Autodesk Fusion 360 part; units mm, degrees
sketch "Sketch1" plane through (0, 0, 0) normal (0, 0, 1) x (1, 0, 0)
  line L0 (-12.2461, -1.8602) -> (-7.8071, 9.2886)
  line L1 (-7.8071, 9.2886) -> (4.0675, 11.0187)
  line L2 (4.0675, 11.0187) -> (11.5031, 1.6)
  line L3 (11.5031, 1.6) -> (7.0641, -9.5488)
  line L4 (7.0641, -9.5488) -> (-4.8105, -11.2789)
  line L5 (-4.8105, -11.2789) -> (-12.2461, -1.8602)
  line L6 (-4.8105, -11.2789) -> (7.0641, -9.5488)
  line L7 (7.0641, -9.5488) -> (9.515, -26.3712)
  line L8 (9.515, -26.3712) -> (-2.3596, -28.1013)
  line L9 (-2.3596, -28.1013) -> (-4.8105, -11.2789)
  line L10 (7.0641, -9.5488) -> (11.5031, 1.6)
  line L11 (11.5031, 1.6) -> (27.2972, -4.6887)
  line L12 (27.2972, -4.6887) -> (22.8582, -15.8374)
  line L13 (22.8582, -15.8374) -> (7.0641, -9.5488)
  line L14 (11.5031, 1.6) -> (4.0675, 11.0187)
  line L15 (4.0675, 11.0187) -> (17.4107, 21.5524)
  line L16 (17.4107, 21.5524) -> (24.8463, 12.1337)
  line L17 (24.8463, 12.1337) -> (11.5031, 1.6)
  line L18 (4.0675, 11.0187) -> (-7.8071, 9.2886)
  line L19 (-7.8071, 9.2886) -> (-10.258, 26.111)
  line L20 (-10.258, 26.111) -> (1.6166, 27.841)
  line L21 (1.6166, 27.841) -> (4.0675, 11.0187)
  line L22 (-7.8071, 9.2886) -> (-12.2461, -1.8602)
  line L23 (-12.2461, -1.8602) -> (-28.0402, 4.4284)
  line L24 (-28.0402, 4.4284) -> (-23.6012, 15.5772)
  line L25 (-23.6012, 15.5772) -> (-7.8071, 9.2886)
  line L26 (-12.2461, -1.8602) -> (-4.8105, -11.2789)
  line L27 (-4.8105, -11.2789) -> (-18.1537, -21.8127)
  line L28 (-18.1537, -21.8127) -> (-25.5893, -12.394)
  line L29 (-25.5893, -12.394) -> (-12.2461, -1.8602)
  line L30 (-28.0402, 4.4284) -> (-25.5893, -12.394)
  line L31 (-18.1537, -21.8127) -> (-2.3596, -28.1013)
  line L32 (9.515, -26.3712) -> (22.8582, -15.8374)
  line L33 (27.2972, -4.6887) -> (24.8463, 12.1337)
  line L34 (17.4107, 21.5524) -> (1.6166, 27.841)
  line L35 (-10.258, 26.111) -> (-23.6012, 15.5772)
  line L36 (-33.1811, 5.0333) -> (-27.7509, 18.6715)
  line L37 (-12.3047, 30.8656) -> (-27.7509, 18.6715)
  line L38 (-12.3047, 30.8656) -> (2.2215, 32.982)
  line L39 (20.505, 25.7021) -> (2.2215, 32.982)
  line L40 (20.505, 25.7021) -> (29.6009, 14.1803)
  line L41 (32.4381, -5.2936) -> (29.6009, 14.1803)
  line L42 (32.4381, -5.2936) -> (27.0079, -18.9317)
  line L43 (11.5616, -31.1258) -> (27.0079, -18.9317)
  line L44 (11.5616, -31.1258) -> (-2.9645, -33.2422)
  line L45 (-21.248, -25.9624) -> (-2.9645, -33.2422)
  line L46 (-21.248, -25.9624) -> (-30.3439, -14.4406)
  line L47 (-33.1811, 5.0333) -> (-30.3439, -14.4406)
  dimension "d1" = 12
  dimension "d2" = 12
  dimension "d3" = 12
  dimension "d4" = 12
  dimension "d5" = 12
  dimension "d6" = 12
  dimension "d7" = 120
  dimension "d8" = 120
  dimension "d9" = 120
  dimension "d10" = 17
  dimension "d11" = 17
  dimension "d12" = 17
  dimension "d13" = 17
  dimension "d14" = 17
  dimension "d15" = 17
  dimension "d16" = -5
extrude "Extrude1" add sketch "Sketch1" along normal blind 3
sketch "Sketch2" plane through (0, 0, 0) normal (0, 0, -1) x (1, 0, 0)
  line L0 (17.4107, -21.5524) -> (1.6166, -27.841)
  line L1 (1.6166, -27.841) -> (-10.258, -26.111)
  line L2 (-10.258, -26.111) -> (-23.6012, -15.5772)
  line L3 (-23.6012, -15.5772) -> (-28.0402, -4.4284)
  line L4 (-28.0402, -4.4284) -> (-25.5893, 12.394)
  line L5 (-25.5893, 12.394) -> (-18.1537, 21.8127)
  line L6 (-18.1537, 21.8127) -> (-2.3596, 28.1013)
  line L7 (-2.3596, 28.1013) -> (9.515, 26.3712)
  line L8 (9.515, 26.3712) -> (22.8582, 15.8374)
  line L9 (22.8582, 15.8374) -> (27.2972, 4.6887)
  line L10 (27.2972, 4.6887) -> (24.8463, -12.1337)
  line L11 (24.8463, -12.1337) -> (17.4107, -21.5524)
  line L12 (-27.7509, -18.6715) -> (-12.3047, -30.8656)
  line L13 (-12.3047, -30.8656) -> (2.2215, -32.982)
  line L14 (2.2215, -32.982) -> (20.505, -25.7021)
  line L15 (20.505, -25.7021) -> (29.6009, -14.1803)
  line L16 (29.6009, -14.1803) -> (32.4381, 5.2936)
  line L17 (32.4381, 5.2936) -> (27.0079, 18.9317)
  line L18 (27.0079, 18.9317) -> (11.5616, 31.1258)
  line L19 (11.5616, 31.1258) -> (-2.9645, 33.2422)
  line L20 (-2.9645, 33.2422) -> (-21.248, 25.9624)
  line L21 (-21.248, 25.9624) -> (-30.3439, 14.4406)
  line L22 (-30.3439, 14.4406) -> (-33.1811, -5.0333)
  line L23 (-33.1811, -5.0333) -> (-27.7509, -18.6715)
  line L24 (-30.3439, 14.4406) -> (-33.1811, -5.0333)
  line L25 (-30.2125, -5.4658) -> (-27.3752, 14.0081)
  line L26 (-10.4458, -28.5109) -> (-25.892, -16.3168)
  line L27 (-27.7509, -18.6715) -> (-12.3047, -30.8656)
  line L28 (19.3952, -22.915) -> (1.1117, -30.1948)
  line L29 (2.2215, -32.982) -> (20.505, -25.7021)
  line L30 (29.4695, 5.7261) -> (26.6322, -13.7478)
  line L31 (29.6009, -14.1803) -> (32.4381, 5.2936)
  line L32 (9.7027, 28.7711) -> (25.149, 16.5771)
  line L33 (27.0079, 18.9317) -> (11.5616, 31.1258)
  line L34 (-20.1382, 23.1752) -> (-1.8547, 30.455)
  line L35 (-2.9645, 33.2422) -> (-21.248, 25.9624)
  line L36 (-20.1382, 23.1752) -> (-27.3752, 14.0081)
  line L37 (-30.2125, -5.4658) -> (-25.892, -16.3168)
  line L38 (-10.4458, -28.5109) -> (1.1117, -30.1948)
  line L39 (19.3952, -22.915) -> (26.6322, -13.7478)
  line L40 (29.4695, 5.7261) -> (25.149, 16.5771)
  line L41 (9.7027, 28.7711) -> (-1.8547, 30.455)
  line L42 (-30.3439, 14.4406) -> (-21.248, 25.9624)
  line L43 (-2.9645, 33.2422) -> (11.5616, 31.1258)
  line L44 (27.0079, 18.9317) -> (32.4381, 5.2936)
  line L45 (29.4695, -14.3468) -> (20.505, -25.7021)
  line L46 (2.2215, -32.982) -> (-12.3047, -30.8656)
  line L47 (-27.7509, -18.6715) -> (-33.1811, -5.0333)
  dimension "d20" = 2
extrude "Extrude2" add sketch "Sketch2" along normal blind 5 contours L12 L13 L14 L15 L16 L17 L18 L19 L20 L21 L22 L23 L24 L27 L29 L31 L33 L35 L42 L43 L44 L45 L46 L47
sketch "Sketch3" plane through (17.718, -22.4435, 0) normal (-0.6196, 0.7849, 0) x (-0.7849, -0.6196, 0)
  line L0 (10.212, 0) -> (-9.4675, 0)
  line L1 (-9.4675, 0) -> (-9.4675, -5)
  line L2 (-9.4675, -5) -> (10.212, -5)
  line L3 (10.212, -5) -> (10.212, 0)
  line L4 (1.005, -5) -> (-0.2606, -5)
  line L5 (-0.2606, -5) -> (-0.2606, -3.2743)
  line L6 (1.005, -3.2743) -> (1.005, -5)
  arc A0 (1.005, -3.2743) -> (-0.2606, -3.2743) centre (0.3722, -2.5) ccw
  point P0 (0.3722, -2.5)
  dimension "d25" = 2
extrude "Extrude3" cut sketch "Sketch3" against normal blind 7 contours L2 L4 L5 L6 A0
pattern_circular "C-Pattern1" count 6 over 360 about axis through (-0.3715, -0.1301, 1) along (0, 0, -1) of "Extrude3"
Verification items for the finished model (mm, model axes). A direction names the side the tool comes from. Give positions to 0.01 mm unless a question says otherwise; leave off trailing zeros. Loops run counter-clockwise (first coordinate to the right, second up) from the corner with the lowest first, then second, coordinate; pieces in that order, holes last. Notation, with made-up numbers: M 18,66.5 L 32,66.5 A8 cw 32,71.5 Z; hole C 6,-8.75 d2. An arc over 180 degrees is marked long. One line per question, with ' | ' between items.
Item 1: Section check C-C, the plane x = -15. Record the cut outline in (y, z).
Completed:
outline: M -28.45,-5 L -25.22,-5 L -25.22,0 L -23.07,0 L -23.07,3 L -28.45,3 Z; M 22.37,0 L 24.92,0 L 24.92,-5 L 28.74,-5 L 28.74,3 L 22.37,3 Z
Item 2: Section check A-A, the plane z = 1.25. Record the cut outline in (x, y) (1 decimal), plus the area to 3 significant figures.
Completed:
outline: M -33.2,5 L -30.3,-14.4 L -21.2,-26 L -3,-33.2 L 11.6,-31.1 L 27,-18.9 L 32.4,-5.3 L 29.6,14.2 L 20.5,25.7 L 2.2,33 L -12.3,30.9 L -27.8,18.7 Z; hole M -28,4.4 L -25.6,-12.4 L -18.2,-21.8 L -2.4,-28.1 L 9.5,-26.4 L 22.9,-15.8 L 27.3,-4.7 L 24.8,12.1 L 17.4,21.6 L 1.6,27.8 L -10.3,26.1 L -23.6,15.6 Z | area: 950 mm^2
Item 3: Draft check along Y on faces 6 (the face through (16.09, -21.18, 1.48)), 7 (the face through (19.18, -25.11, -1.06)), 8 (the face through (10.8, 27.9, -1.5)), 9 (the face through (11.49, 29.29, -1.06)). Enter one of: +Y half, -Y half, draft (parallel to the pull), parting line (faces both ways), or undercut.
Completed:
face 6: undercut | face 7: -Y half | face 8: undercut | face 9: +Y half
Item 4: Section check B-B, the plane y = -21. Record the cut outline in (x, z), plus the area to 3 significant figures.
Completed:
outline: M -25.17,-5 L -21.86,-5 L -21.86,0 L -18.8,0 L -18.8,3 L -25.17,3 Z; M 16.32,0 L 19.55,0 L 19.55,-5 L 24.39,-5 L 24.39,3 L 16.32,3 Z | area: 84.1 mm^2
Item 5: Depth check by flat-ended pin: P1, Ø2, axis at y = 17, z = -0.5, coming from the -X side; P2, Ø4, axis at y = 6.5, z = -1, coming from the +X side; P3, Ø2, axis at y = 21, z = 0.5, coming from the +X side. Enter the tip coordinate at first touch or a pass-through.
Completed:
P1: stops at x = -28.81 | P2: stops at x = 31.01 | P3: stops at x = 25.01
Item 6: Tool access check on faces 1 (the face through (25.109, -10.185, 1.479)), 2 (the face through (24.99, 20.02, -1.06)), 3 (the face through (28.07, 3.87, -1.35)), 4 (the face through (29.42, 4.85, -4.15)), 5 (the face through (-30.17, -5.11, -4.15)). Record the directions out of +Z, -Z, +X, -X, +Y, -Y that give a thin tool (end or side, any length) a straight path to the whole face; none if there is none.
Completed:
face 1: +Z, -Z | face 2: +Z, -Z, +X, +Y | face 3: -Z | face 4: -Z, +X | face 5: -Z, -X
Item 7: Thickness scan on line 1 (Z direction, x = 10.5, y = 26); line 2 (Y direction, x = -16.5, z = 0.5); line 3 (Y direction, x = -5.5, z = -2). Record the ranges inside material, lowest first. Write a range as [from, to].
Completed:
line 1: z = [0, 3] | line 2: y = [-27.85, -22.47], [21.18, 27.55] | line 3: y = [-32.23, -29], [29.23, 31.86]
